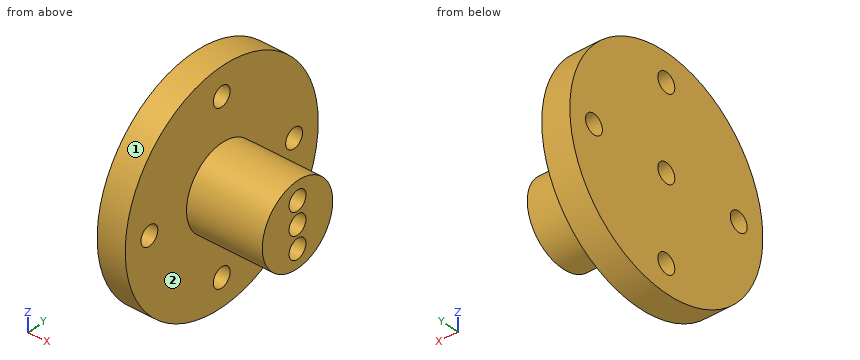
Autodesk Inventor part; units mm, degrees
ref_plane "YZ Plane" through (0, 0, 0) normal (1, 0, 0) x (0, 1, 0)
ref_plane "XZ Plane" through (0, 0, 0) normal (0, 1, 0) x (-1, 0, 0)
ref_plane "XY Plane" through (0, 0, 0) normal (0, 0, 1) x (1, 0, 0)
sketch "Sketch1" plane through (0, 0, 0) normal (1, 0, 0) x (0, 1, 0)
  circle A0 centre (0, 0) radius 15
  circle A1 centre (15, 0) radius 1.75
  circle A2 centre (0, 15) radius 1.75
  circle A3 centre (-15, 0) radius 1.75
  circle A4 centre (0, -15) radius 1.75
  circle A5 centre (0, 0) radius 1.75
  circle A6 centre (0, 0) radius 20
  dimension "d0" = 30
  dimension "d1" = 3.5
  dimension "d4" = 360
  dimension "d6" = 3.5
  dimension "d7" = 40
extrude "Extrusion1" add sketch "Sketch1" along normal blind 5 contours A1 A0 A4 A3 A2 | A6
sketch "Sketch5" plane through (5, 0, 0) normal (1, 0, 0) x (0, 0, -1)
  circle A0 centre (0, 0) radius 1.75
  circle A1 centre (0, 0) radius 4
  circle A2 centre (4, 0) radius 1.75
  circle A3 centre (-4, 0) radius 1.75
  circle A4 centre (0, 0) radius 7.3
  dimension "d38" = 8
  dimension "d39" = 3.5
  dimension "d42" = 360
  dimension "d44" = 14.6
extrude "Extrusion5" add sketch "Sketch5" along normal blind 13.5 contours A2 A1 A3 | A4
equation "\"BendRadius\" = Thickness"
equation "\"BendReliefWidth\" = Thickness"
equation "\"BendReliefDepth\" = 0.5 * Thickness"
equation "\"CornerReliefSize\" = 4 * Thickness"
equation "\"MinimumRemnant\" = 2 * Thickness"
equation "\"TransitionRadius\" = BendRadius"
equation "\"JacobiRadiusSize\" = BendRadius"
equation "\"GapSize\" = Thickness"
properties part number "EaglePowerCycDriveAdaptor"
The listing builds one solid part. Answer for the finished solid, in the listing's coordinates (mm). Face numbers are marked on the shaded views. A direction names the side the tool comes from. Give positions to 0.01 mm unless a question says otherwise; leave off trailing zeros. Loops run counter-clockwise (first coordinate to the right, second up) from the corner with the lowest first, then second, coordinate; pieces in that order, holes last. Notation, with made-up numbers: (84, -23.5) - (136, -23.5) arc R18 cw to (136, 7.5) - close; hole circle Ø9 at (20.25, 30). An arc over 180 degrees is marked (long way). Answer as a JSON object with one key per item and string values.
1. A cutting plane is placed at D-D (x = 3). Write down the section's boundary in (y, z), then the cut area to 3 significant figures.
Determined:
{"outline": "circle Ø40 at (0, 0); hole circle Ø3.5 at (-15, 0); hole circle Ø3.5 at (0, -15); hole circle Ø3.5 at (0, 0); hole circle Ø3.5 at (0, 15); hole circle Ø3.5 at (15, 0)", "area": "1,210 mm²"}
2. A cutting plane is placed at A-A (y = 0). Write down the section's boundary in (x, z), then the cut area to 3 significant figures.
Determined:
{"outline": "(0, -20) - (5, -20) - (5, -16.75) - (0, -16.75) - close; (0, -13.25) - (5, -13.25) - (5, -7.3) - (18.5, -7.3) - (18.5, -5.75) - (5, -5.75) - (5, -2.25) - (18.5, -2.25) - (18.5, -1.75) - (0, -1.75) - close; (0, 1.75) - (18.5, 1.75) - (18.5, 2.25) - (5, 2.25) - (5, 5.75) - (18.5, 5.75) - (18.5, 7.3) - (5, 7.3) - (5, 13.25) - (0, 13.25) - close; (0, 16.75) - (5, 16.75) - (5, 20) - (0, 20) - close", "area": "203 mm²"}
3. A cutting plane is placed at C-C (z = -14). Write down the section's boundary in (x, y), then the cut area to 3 significant figures.
Determined:
{"outline": "(0, -14.28) - (5, -14.28) - (5, -1.44) - (0, -1.44) - close; (0, 1.44) - (5, 1.44) - (5, 14.28) - (0, 14.28) - close", "area": "128 mm²"}
4. A cutting plane is placed at B-B (y = 14.5). Write down the section's boundary in (x, z).
Determined:
{"outline": "(0, -13.77) - (5, -13.77) - (5, -1.68) - (0, -1.68) - close; (0, 1.68) - (5, 1.68) - (5, 13.77) - (0, 13.77) - close"}
5. Flat-ended cylindrical pins translate along their axes: pin 1 Ø3 at (y, z) = (-15, 0) entering from -X; pin 2 Ø5 at (x, y) = (7, 2) entering from +Z; pin 3 Ø3 at (y, z) = (0, 4) entering from +X; pin 4 Ø10 at (x, y) = (8, 3) entering from -Z. Find the tip coordinate at first contact, or state that the pin passes through.
Determined:
{"pin 1": "through", "pin 2": "z = 19.99", "pin 3": "x = 5", "pin 4": "z = -20"}
6. Find the intervals of material crossed by L1, parallel to Y at x = 12.75, z = 0; L2, parallel to X at y = -6, z = -5; L3, parallel to Y at x = 2.35, z = 15, in increasing order. Write a range as [from, to].
Determined:
{"L1": "[-7.3, -1.75], [1.75, 7.3]", "L2": "[0, 5]", "L3": "[-13.23, -1.75], [1.75, 13.23]"}
7. For the marked faces 1 and 2, determine the directions among +Z, -Z, +X, -X, +Y, -Y from which every point of the face is accessible in a straight line to the end or side of a thin tool.
Determined:
{"face 1": "+X, -X", "face 2": "+X"}
